```python
from build123d import *

# Parameters (mm, degrees)
SKETCH_1_R          = 70
SKETCH_1_R_2        = 57.5
EXTRUDE_1_DEPTH     = 8.6
SKETCH_2_R          = 2.5
CUT_EXTRUDE_1_DEPTH = 100.367801626
CHAMFER_1_SIZE      = 0.5
SKETCH_3_R          = 1.65
CUT_EXTRUDE_2_DEPTH = 100.367801626
SKETCH_4_R          = 1.6
CUT_EXTRUDE_3_DEPTH = 100.367801626


with BuildPart() as part:
    # ｽｹｯﾁ1 → ﾎﾞｽ - 押し出し1 (new body)
    with BuildSketch(Plane(origin=(0, 0, 0), x_dir=(1, 0, 0), z_dir=(0, 1, 0))):
        with Locations(Location((0, 0, 0), (0, 0, 90))):
            Circle(SKETCH_1_R)
        with Locations(Location((0, 0, 0), (0, 0, 90))):
            Circle(SKETCH_1_R_2, mode=Mode.SUBTRACT)
    extrude(amount=EXTRUDE_1_DEPTH)

    # ｽｹｯﾁ2 → ｶｯﾄ - 押し出し1 (cut, through all)
    with BuildSketch(Plane(origin=(0, 8.6, 0), x_dir=(1, 0, 0), z_dir=(0, 1, 0))):
        with Locations(Location((-44.72450391, 44.72450391, 0), (0, 0, 270))):
            Circle(SKETCH_2_R)
        with Locations(Location((44.72450391, 44.72450391, 0), (0, 0, 270))):
            Circle(SKETCH_2_R)
        with Locations(Location((44.72450391, -44.72450391, 0), (0, 0, 270))):
            Circle(SKETCH_2_R)
        with Locations(Location((-44.72450391, -44.72450391, 0), (0, 0, 270))):
            Circle(SKETCH_2_R)
    extrude(amount=-CUT_EXTRUDE_1_DEPTH, mode=Mode.SUBTRACT)

    # 面取り1
    chamfer_1_edges = [part.edges().sort_by_distance(p)[0] for p in [
        (0, 0, 70),
        (0, 8.6, 70),
        (0, 0, 57.5),
        (0, 8.6, 57.5),
    ]]
    chamfer(chamfer_1_edges, length=CHAMFER_1_SIZE)

    # ｽｹｯﾁ3 → ｶｯﾄ - 押し出し2 (cut, through all)
    with BuildSketch(Plane(origin=(0, 8.6, 0), x_dir=(1, 0, 0), z_dir=(0, 1, 0))):
        with Locations(Location((65, 0, 0), (0, 0, 270))):
            Circle(SKETCH_3_R)
        with Locations(Location((0, -65, 0), (0, 0, 270))):
            Circle(SKETCH_3_R)
        with Locations(Location((-65, 0, 0), (0, 0, 270))):
            Circle(SKETCH_3_R)
        with Locations(Location((0, 65, 0), (0, 0, 270))):
            Circle(SKETCH_3_R)
        with Locations(Location((-62.5, 20, 0), (0, 0, 270))):
            Circle(SKETCH_3_R)
        with Locations(Location((62.5, 20, 0), (0, 0, 270))):
            Circle(SKETCH_3_R)
        with Locations(Location((62.5, -20, 0), (0, 0, 270))):
            Circle(SKETCH_3_R)
        with Locations(Location((-62.5, -20, 0), (0, 0, 270))):
            Circle(SKETCH_3_R)
    extrude(amount=-CUT_EXTRUDE_2_DEPTH, mode=Mode.SUBTRACT)

    # ｽｹｯﾁ4 → ｶｯﾄ - 押し出し3 (cut, through all)
    with BuildSketch(Plane(origin=(0, 8.6, 0), x_dir=(1, 0, 0), z_dir=(0, 1, 0))):
        with Locations(Location((51.567967119, 39.569492886, 0), (0, 0, 270))):
            Circle(SKETCH_4_R)
        with Locations(Location((39.569492886, 51.567967119, 0), (0, 0, 270))):
            Circle(SKETCH_4_R)
        with Locations(Location((-39.569492886, 51.567967119, 0), (0, 0, 270))):
            Circle(SKETCH_4_R)
        with Locations(Location((-51.567967119, 39.569492886, 0), (0, 0, 270))):
            Circle(SKETCH_4_R)
    extrude(amount=-CUT_EXTRUDE_3_DEPTH, mode=Mode.SUBTRACT)


solid = part.part
```
CAD build for the part. Positions are in the model's coordinates, mm. Round coordinates to 2 decimals unless told otherwise and drop trailing zeros. Order: outer loops, then holes, each group sorted by start corner. A loop starts at its lowest first (then second) coordinate and runs counter-clockwise, first axis right, second up.
Item 1: Saw through at A-A on z = 0. Write the cut outline in (x, y).
Item 2: Saw through at B-B on x = 0. Write the cut outline in (y, z).
Item 3: Probe line 1 along X through (y, z) = (1.25, -45); line 2 along X through (y, z) = (5, -18.5); line 3 along Z through (x, y) = (52.5, 2.25). List the from-to ranges inside material, lowest first.
Item 4: Pin check, flat tips, straight feed: pin 1 (2 mm diameter, centred on x = 10.5, y = 1, fed in from +Z); pin 2 (3 mm diameter, centred on x = -37, y = 6.5, fed in from -Z); pin 3 (2 mm diameter, centred on y = 4.5, z = -22.5, fed in from +X). Stop position of each tip, or through.
Item 5: Saw through at C-C on y = 3. State how many separate pieces and enclosed holes the cut face has, then the cut area to 3 significant figures.
Item 6: Mould opens along X. For faces 1 (the face through (41, 8.6, 42)), 2 (the face through (42.594, 4.247, 55.55)), 3 (the face through (42.284, 4.36, -45.266)) say: pulls with the +X half, pulls with the -X half, needs draft (parallel to the pull), parting line crosses it, or undercut.
Reported:
1. outline: (-70, 0.5) - (-69.5, 0) - (-66.65, 0) - (-66.65, 8.6) - (-69.5, 8.6) - (-70, 8.1) - close; (-63.35, 0) - (-58, 0) - (-57.5, 0.5) - (-57.5, 8.1) - (-58, 8.6) - (-63.35, 8.6) - close; (57.5, 0.5) - (58, 0) - (63.35, 0) - (63.35, 8.6) - (58, 8.6) - (57.5, 8.1) - close; (66.65, 0) - (69.5, 0) - (70, 0.5) - (70, 8.1) - (69.5, 8.6) - (66.65, 8.6) - close
2. outline: (0, -69.5) - (0.5, -70) - (8.1, -70) - (8.6, -69.5) - (8.6, -66.65) - (0, -66.65) - close; (0, -63.35) - (8.6, -63.35) - (8.6, -58) - (8.1, -57.5) - (0.5, -57.5) - (0, -58) - close; (0, 58) - (0.5, 57.5) - (8.1, 57.5) - (8.6, 58) - (8.6, 63.35) - (0, 63.35) - close; (0, 66.65) - (8.6, 66.65) - (8.6, 69.5) - (8.1, 70) - (0.5, 70) - (0, 69.5) - close
3. line 1: x = -53.62 to -47.21, -42.24 to -35.79, 35.79 to 42.24, 47.21 to 53.62
3. line 2: x = -67.51 to -63.19, -61.81 to -54.44, 54.44 to 61.81, 63.19 to 67.51
3. line 3: z = -46.3 to -40.87, -38.27 to -23.45, 23.45 to 46.3
4. pin 1: stops at z = 69.35
4. pin 2: stops at z = -60.33
4. pin 3: stops at x = 66.62
5. separate pieces: 1
5. enclosed holes: 17
5. area: 4,830 mm2
6. face 1: needs draft
6. face 2: parting line crosses it
6. face 3: undercut
